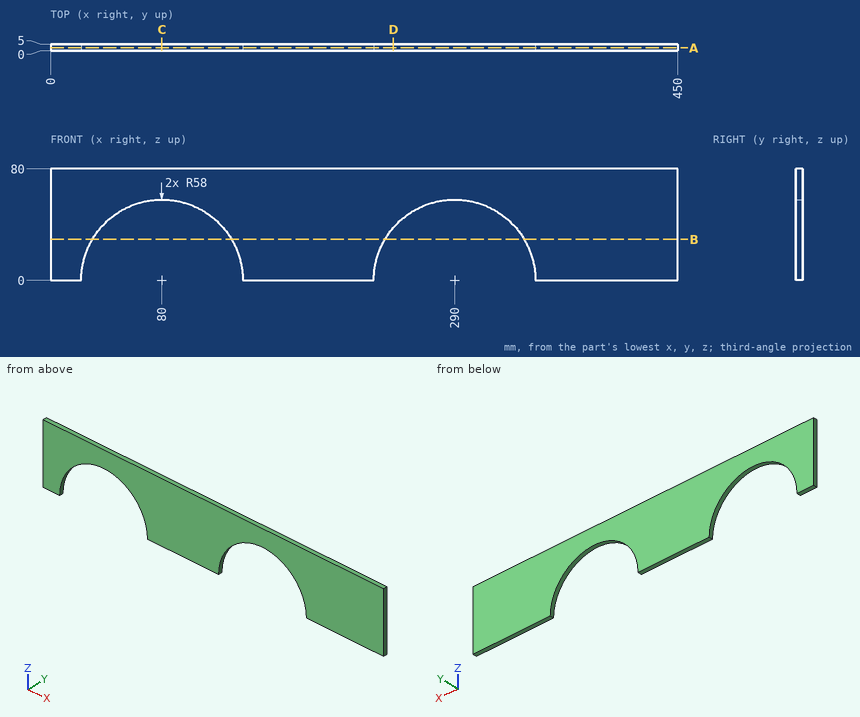
Could you check a few things on this drawing? It's one solid part, dimensions in mm from its lowest x, y, z. Round coordinates to 2 decimals unless told otherwise and drop trailing zeros. Order: outer loops, then holes, each group sorted by start corner. A loop starts at its lowest first (then second) coordinate and runs counter-clockwise, first axis right, second up. Notation, with made-up numbers: (-3, 9.5) -> (25, 9.5) arc R19 ccw to (25, 16.5) -> close; hole circle Ø10 at (-18, -7.75). An arc over 180 degrees is marked (long way). One line per question, with ' | ' between items.
Q1. If I drill on line 1 (X direction, y = 3.9, z = 31.5); line 2 (X direction, y = 2.3, z = 29); line 3 (Z direction, x = 77, y = 2), over which ranges is the centre line in solid material (lowest first)? Write a range as from..to.
Computed values:
line 1: 0..31.3, 128.7..241.3, 338.7..450 | line 2: 0..29.77, 130.23..239.77, 340.23..450 | line 3: 57.92..80
Q2. If we section it at D-D on x = 246: Write out the boundary of the cut face in (y, z), plus the area to 3 significant figures.
Computed values:
outline: (0, 37.79) -> (5, 37.79) -> (5, 80) -> (0, 80) -> close | area: 211 mm²
Q3. If we section it at B-B on z = 29.5: Write out the boundary of the cut face in (x, y), plus the area to 3 significant figures.
Computed values:
outline: (0, 0) -> (30.06, 0) -> (30.06, 5) -> (0, 5) -> close; (129.94, 0) -> (240.06, 0) -> (240.06, 5) -> (129.94, 5) -> close; (339.94, 0) -> (450, 0) -> (450, 5) -> (339.94, 5) -> close | area: 1,250 mm²
Q4. If we section it at C-C on x = 80: Write out the boundary of the cut face in (y, z).
Computed values:
outline: (0, 58) -> (5, 58) -> (5, 80) -> (0, 80) -> close
Q5. If we section it at A-A on y = 2.3: Write out the boundary of the cut face in (x, z), plus the area to 3 significant figures.
Computed values:
outline: (0, 0) -> (22, 0) arc R58 cw to (138, 0) -> (232, 0) arc R58 cw to (348, 0) -> (450, 0) -> (450, 80) -> (0, 80) -> close | area: 25,400 mm²
